Geometry check sheet. Reference: the model listing, model coordinates, mm. Face numbers are marked on the shaded views. A direction names the side the tool comes from. Round coordinates to 2 decimals unless told otherwise and drop trailing zeros. Write each loop counter-clockwise with the first axis right and the second up, starting at its lowest first coordinate (ties: lowest second). Pieces come first, ordered by that corner, then holes. Notation, with made-up numbers: (-32, 40.25) -> (11, 40.25) arc R31 cw to (11, 79.25) -> close; hole circle Ø1 at (73, 8.25). An arc over 180 degrees is marked (long way). Return JSON: item names as keys, results as strings. Group by question number.
from build123d import *

# Parameters (mm, degrees)
F0_W     = 10.62
F0_H     = 12.65
F1_DEPTH = 10.16
F3_DEPTH = 2.54
F4_DEPTH = 2.54
F5_DEPTH = 2.54
F6_DEPTH = 2.54
F7_DEPTH = 2.54
F8_DEPTH = 2.54


with BuildPart() as f1:
    # F0 (on Top) → F1 (new body)
    with BuildSketch(Plane.XY):
        Polygon((50.799853, -0.122195), (25.505751, 43.932866), (-25.294102, 44.055061), (-50.799853, 0.122195), (-25.505751, -43.932866), (25.294102, -44.055061), align=None)
        Polygon((-3.33668, -25.740905), (3.511563, -25.896048), (6.801327, -31.904372), (3.242847, -37.757553), (-3.605395, -37.60241), (-6.895159, -31.594086), align=None, mode=Mode.SUBTRACT)
        Polygon((-24.849274, -7.47878), (-21.448886, -13.43441), (-24.906419, -19.357047), (-31.76434, -19.324054), (-35.164728, -13.368424), (-31.707195, -7.445787), align=None, mode=Mode.SUBTRACT)
        Polygon((23.739571, -20.126873), (20.339183, -14.171243), (23.796716, -8.248606), (30.654636, -8.281598), (34.055024, -14.237228), (30.597491, -20.159865), align=None, mode=Mode.SUBTRACT)
        Polygon((-21.384008, 13.537441), (-24.813008, 7.598239), (-31.671008, 7.598239), (-35.100008, 13.537441), (-31.671008, 19.476643), (-24.813008, 19.476643), align=None, mode=Mode.SUBTRACT)
        Rectangle(F0_W, F0_H, mode=Mode.SUBTRACT)
        Polygon((34.123123, 14.07323), (30.694123, 8.134028), (23.836123, 8.134028), (20.407123, 14.07323), (23.836123, 20.012433), (30.694123, 20.012433), align=None, mode=Mode.SUBTRACT)
        Polygon((-6.743086, 31.626892), (-3.424455, 37.61932), (3.424455, 37.741515), (6.954734, 31.871283), (3.636104, 25.878855), (-3.212806, 25.75666), align=None, mode=Mode.SUBTRACT)
    extrude(amount=F1_DEPTH)

    # F2 (on face) → F3 (join)
    with BuildSketch(Plane(origin=(0, 0, 0), x_dir=(1, 0, 0), z_dir=(0, 0, -1))):
        Polygon((44.630353, 0.201512), (22.489691, -38.550264), (23.831054, -41.276596), (47.662108, 0), align=None)
    extrude(amount=F3_DEPTH)

    # F2 (on face) → F4 (join)
    with BuildSketch(Plane(origin=(0, 0, 0), x_dir=(1, 0, 0), z_dir=(0, 0, -1))):
        Polygon((22.140662, 38.751775), (44.630353, 0.201512), (47.662108, 0), (23.831054, 41.276596), align=None)
    extrude(amount=F4_DEPTH)

    # F2 (on face) → F5 (join)
    with BuildSketch(Plane(origin=(0, 0, 0), x_dir=(1, 0, 0), z_dir=(0, 0, -1))):
        Polygon((-23.831054, 41.276596), (-22.489691, 38.550264), (22.140662, 38.751775), (23.831054, 41.276596), align=None)
    extrude(amount=F5_DEPTH)

    # F2 (on face) → F6 (join)
    with BuildSketch(Plane(origin=(0, 0, 0), x_dir=(1, 0, 0), z_dir=(0, 0, -1))):
        Polygon((-47.662108, 0), (-44.630353, -0.201512), (-22.489691, 38.550264), (-23.831054, 41.276596), align=None)
    extrude(amount=F6_DEPTH)

    # F2 (on face) → F7 (join)
    with BuildSketch(Plane(origin=(0, 0, 0), x_dir=(1, 0, 0), z_dir=(0, 0, -1))):
        Polygon((-23.831054, -41.276596), (-22.140662, -38.751775), (-44.630353, -0.201512), (-47.662108, 0), align=None)
    extrude(amount=F7_DEPTH)

    # F2 (on face) → F8 (join)
    with BuildSketch(Plane(origin=(0, 0, 0), x_dir=(1, 0, 0), z_dir=(0, 0, -1))):
        Polygon((22.489691, -38.550264), (-22.140662, -38.751775), (-23.831054, -41.276596), (23.831054, -41.276596), align=None)
    extrude(amount=F8_DEPTH)


solid = f1.part
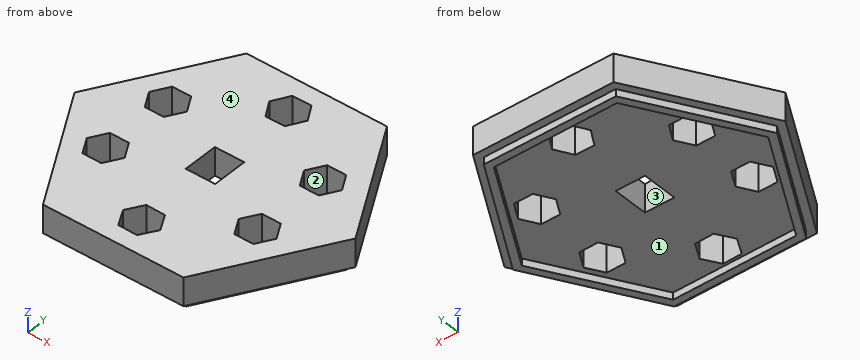
1) Sectioned sample at C-C on z = 8.75. State how many separate pieces and enclosed holes the cut face has, and give its area (3 significant figures).
2) Sectioned sample at A-A on y = -36. Enter the section's corners in (x, z), and give its area (3 significant figures).
3) Sectioned sample at D-D on y = 27.5. Enter the section's corners in (x, z).
4) Go/stop test with flat-tipped pins: P1, Ø5.5, axis at x = 26.5, z = 3, coming from the +Y side; P2, Ø1.5, axis at y = 15.5, z = 8.5, coming from the +X side; P3, Ø1, axis at y = -2, z = 5.5, coming from the -X side. Record where each tip stops, or that it passes through.
5) Material ranges on probe 1 along Y at (x, z) = (21, 0.5); probe 2 along Y at (x, z) = (-4, 6) (3 decimals); probe 3 along X at (y, z) = (19, 1), recorded low to high. Write a range as [from, to].
6) Mould release check, pull along X, two halves, no side actions. Record for the marked faces 3 and 4: +X half, -X half, draft (parallel to the pull), parting line (faces both ways), or undercut.
7) Tool access check on the marked faces 1 and 2. Record the directions out of +Z, -Z, +X, -X, +Y, -Y that give a thin tool (end or side, any length) a straight path to the whole face; none if there is none.
8) Sectioned sample at B-B on x = -1.5. Enter the section's corners in (y, z) (3 decimals), and give its area (3 significant figures).
Evaluation:
{
 "1": {"separate pieces": "1", "enclosed holes": "7", "area": "5,840 mm2"},
 "2": {"outline": "(-30.06, 0) -> (-26.88, 0) -> (-26.88, -2.54) -> (-23.95, -2.54) -> (-23.95, 0) -> (-4.48, 0) -> (-4.48, 10.16) -> (-30.06, 10.16) -> close; (4.31, 0) -> (23.75, 0) -> (23.75, -2.54) -> (26.88, -2.54) -> (26.88, 0) -> (29.97, 0) -> (29.97, 10.16) -> (4.31, 10.16) -> close", "area": "536 mm2"},
 "3": {"outline": "(-34.91, 0) -> (-31.78, 0) -> (-31.78, -2.54) -> (-28.7, -2.54) -> (-28.7, 0) -> (-4.26, 0) -> (-4.26, 10.16) -> (-34.91, 10.16) -> close; (4.53, 0) -> (28.8, 0) -> (28.8, -2.54) -> (31.78, -2.54) -> (31.78, 0) -> (34.94, 0) -> (34.94, 10.16) -> (4.53, 10.16) -> close"},
 "4": {"P1": "stops at y = 43.94", "P2": "stops at x = 42.26", "P3": "stops at x = -49.87"},
 "5": {"probe 1": "y = [-44.04, -15.33], [-13.04, 13.05], [15.1, 43.94]", "probe 2": "y = [-43.985, -36.882], [-26.832, -6.325], [6.325, 27.066], [36.58, 44.004]", "probe 3": "x = [-39.84, -31.95], [-24.54, 23.25], [31.28, 39.82]"},
 "6": {"face 3": "undercut", "face 4": "draft"},
 "7": {"face 1": "-Z", "face 2": "+Z, -Z"},
 "8": {"outline": "(-43.991, 0) -> (-41.277, 0) -> (-41.277, -2.54) -> (-38.645, -2.54) -> (-38.645, 0) -> (-37.65, 0) -> (-37.65, 10.16) -> (-43.991, 10.16) -> close; (-25.783, 0) -> (-6.325, 0) -> (-6.325, 10.16) -> (-25.783, 10.16) -> close; (6.325, 0) -> (25.787, 0) -> (25.787, 10.16) -> (6.325, 10.16) -> close; (37.654, 0) -> (38.659, 0) -> (38.659, -2.54) -> (41.277, -2.54) -> (41.277, 0) -> (43.998, 0) -> (43.998, 10.16) -> (37.654, 10.16) -> close", "area": "538 mm2"}
}
